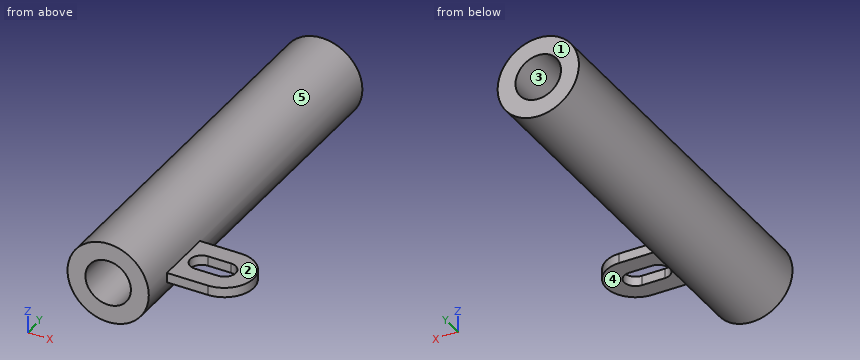
```python
from build123d import *

# Parameters (mm, degrees)
F0_R     = 12.5
F0_R_2   = 7
F1_DEPTH = 58.075
F3_DEPTH = 1.5


with BuildPart() as f1:
    # F0 (on Front) → F1 (new body, symmetric)
    with BuildSketch(Plane.XZ):
        Circle(F0_R)
        Circle(F0_R_2, mode=Mode.SUBTRACT)
    extrude(amount=F1_DEPTH, both=True)

    # F2 (on Top) → F3 (join, symmetric)
    with BuildSketch(Plane.XY):
        with BuildLine():
            Line((10, -30.075), (10, -48.075))
            Line((10, -48.075), (25, -48.075))
            ThreePointArc((25, -48.075), (34, -39.075), (25, -30.075))
            Line((25, -30.075), (10, -30.075))
        make_face()
        with BuildLine():
            Line((18, -35.575), (25, -35.575))
            ThreePointArc((25, -35.575), (28.5, -39.075), (25, -42.575))
            Line((25, -42.575), (18, -42.575))
            ThreePointArc((18, -42.575), (14.5, -39.075), (18, -35.575))
        make_face(mode=Mode.SUBTRACT)
    extrude(amount=F3_DEPTH, both=True)


solid = f1.part
```
Read the model definition and answer for the solid it produces. Units are mm, in the model's axes. Face numbers are marked on the shaded views. A direction names the side the tool comes from. Round coordinates to 2 decimals unless told otherwise and drop trailing zeros. Write each loop counter-clockwise with the first axis right and the second up, starting at its lowest first coordinate (ties: lowest second). Pieces come first, ordered by that corner, then holes. Notation, with made-up numbers: M 69.25,21.5 L 105.25,21.5 A16 ccw 105.25,27.5 Z; hole C 70.5,72.5 d11. An arc over 180 degrees is marked long. One line per item, written item: value.
Q1. Find section C-C on y = -11. Write down the section's boundary in (x, z).
Data:
outline: C 0,0 d25; hole C 0,0 d14
Q2. For a pull along X with two mould halves and no side action, classify the marked faces 3, 4 and 5 as +X half, -X half, draft (parallel to the pull), parting line (faces both ways), or undercut.
Data:
face 3: undercut
face 4: draft
face 5: parting line
Q3. Which of the six approach directions +Z, -Z, +X, -X, +Y, -Y give full straight-line access (tool end or side, diameter ignored) to the marked faces 1 and 2?
Data:
face 1: +Z, -Z, +X, -X, +Y
face 2: +Z, +X, +Y, -Y
Q4. Straight lines are drawn through the part: line 1 (Z direction, x = 0, y = -13); line 2 (Z direction, x = 1.5, y = -6); line 3 (X direction, y = 41, z = -4). For each, find the intervals that lie inside material, in ascending order. Write a range as [from, to].
Data:
line 1: [-12.5, -7], [7, 12.5]
line 2: [-12.41, -6.84], [6.84, 12.41]
line 3: [-11.84, -5.74], [5.74, 11.84]
Q5. Flat-ended cylindrical pins translate along their axes: pin 1 Ø6 at (x, y) = (11.5, 10) entering from -Z; pin 2 Ø2 at (y, z) = (1, 8.5) entering from -X; pin 3 Ø0.9 at (x, z) = (19, 0) entering from +Y (3 decimals). Find the tip coordinate at first contact, or state that the pin passes through.
Data:
pin 1: z = -9.17
pin 2: x = -10
pin 3: y = -30.075
Q6. Find section D-D on x = 8.5. Write down the section's boundary in (y, z) (3 decimals).
Data:
outline: M -58.075,-9.165 L 58.075,-9.165 L 58.075,9.165 L -58.075,9.165 Z
Q7. Find section B-B on x = 0. Write down the section's boundary in (y, z) (3 decimals).
Data:
outline: M -58.075,-12.5 L 58.075,-12.5 L 58.075,-7 L -58.075,-7 Z; M -58.075,7 L 58.075,7 L 58.075,12.5 L -58.075,12.5 Z
Q8. Find section A-A on z = 0. Write down the section's boundary in (x, y) (3 decimals).
Data:
outline: M -12.5,-58.075 L -7,-58.075 L -7,58.075 L -12.5,58.075 Z; M 7,-58.075 L 12.5,-58.075 L 12.5,-48.075 L 25,-48.075 A9 ccw 25,-30.075 L 12.5,-30.075 L 12.5,58.075 L 7,58.075 Z; hole M 18,-42.575 L 25,-42.575 A3.5 ccw 25,-35.575 L 18,-35.575 A3.5 ccw Z
